```python
from build123d import *

# Parameters (mm, degrees)
SKETCH1_W                      = 5
SKETCH1_H                      = 25
BOSS_EXTRUDE1_DEPTH            = 10
BOSS_EXTRUDE2_DEPTH            = 2.5
BOSS_EXTRUDE3_START            = 2.5
BOSS_EXTRUDE3_DEPTH            = 2.5
BOSS_EXTRUDE4_DEPTH            = 5
DRAFT1_ANGLE                   = 60
DRAFT2_ANGLE                   = -10
SKETCH6_W                      = 5
SKETCH6_H                      = 15
SKETCH7_W                      = 5
SKETCH7_H                      = 15
SKETCH8_W                      = 5
SKETCH8_H                      = 25
F_10_0_10_DIAMETER_HOLE1_D     = 10
F_10_0_10_DIAMETER_HOLE1_DEPTH = 23.832037061
FILLET1_R                      = 5
FILLET2_R                      = 20


with BuildPart() as part:
    # Sketch1 → Revolve1 (revolve)
    with BuildSketch(Plane(origin=(0, -7.5, 0), x_dir=(1, 0, 0), z_dir=(0, 1, 0))):
        with Locations((-5.811233855, 90.876419512)):
            Rectangle(SKETCH1_W, SKETCH1_H)
    revolve(axis=Axis((-8.311233855, -7.5, -103.376419512), (0, 0, 1)))

    # Sketch2 → Boss-Extrude1 (add)
    with BuildSketch(Plane(origin=(0, -2.5, 0), x_dir=(1, 0, 0), z_dir=(0, 1, 0))):
        with BuildLine():
            Line((-20.904218066, -4.060593221), (-17.745761276, -10))
            ThreePointArc((-17.745761276, -10), (-16.42436709, -8.86625844), (-15.571850751, -7.348145002))
            Line((-15.571850751, -7.348145002), (-13.235172111, -0.671920317))
            ThreePointArc((-13.235172111, -0.671920317), (-13.124251068, -0.312083076), (-13.040724348, 0.055081199))
            ThreePointArc((-13.040724348, 0.055081199), (-9.034250588, -1.999882688), (-5, 0))
            ThreePointArc((-5, 0), (-1.464466094, 1.464466094), (0, 5))
            Line((0, 5), (0, 35))
            ThreePointArc((0, 35), (-10.533604853, 36.723434751), (-20.057952451, 41.541511272))
            Line((-20.057952451, 41.541511272), (5.197843412, 71.090018979))
            Line((5.197843412, 71.090018979), (8.982632418, 71.090018979))
            Line((8.982632418, 71.090018979), (8.982632418, 78.376419512))
            Line((8.982632418, 78.376419512), (-8.311233855, 78.376419512))
            Line((-8.311233855, 78.376419512), (-41.017367582, 78.376419512))
            Line((-41.017367582, 78.376419512), (-54.819345863, 40.83303933))
            Line((-54.819345863, 40.83303933), (-54.896976862, 16.766177236))
            ThreePointArc((-54.896976862, 16.766177236), (-54.712461515, 16.524099343), (-54.430876141, 16.639673113))
            Line((-54.430876141, 16.639673113), (-49.872077715, 24.477250263))
            Line((-49.872077715, 24.477250263), (-8.967847829, 0.684930874))
            Line((-8.967847829, 0.684930874), (-28.967743782, 0.74944331))
            Line((-28.967743782, 0.74944331), (-28.987601327, -5.406715976))
            ThreePointArc((-28.987601327, -5.406715976), (-28.311946244, -7.932877153), (-26.453503439, -9.772494077))
            Line((-26.453503439, -9.772494077), (-20.904218066, -4.060593221))
        make_face()
    extrude(amount=-BOSS_EXTRUDE1_DEPTH)

    # Sketch3 → Boss-Extrude2 (add)
    with BuildSketch(Plane.XZ.offset(12.5)):
        with BuildLine():
            Line((-20.904218066, 4.060593221), (-17.745761276, 10))
            ThreePointArc((-17.745761276, 10), (-16.42436709, 8.86625844), (-15.571850751, 7.348145002))
            Line((-15.571850751, 7.348145002), (-13.235172111, 0.671920317))
            ThreePointArc((-13.235172111, 0.671920317), (-13.124251068, 0.312083076), (-13.040724348, -0.055081199))
            ThreePointArc((-13.040724348, -0.055081199), (-9.034250588, 1.999882688), (-5, 0))
            ThreePointArc((-5, 0), (-1.464466094, -1.464466094), (0, -5))
            Line((0, -5), (0, -35))
            ThreePointArc((0, -35), (-10.533604853, -36.723434751), (-20.057952451, -41.541511272))
            Line((-20.057952451, -41.541511272), (5.197843412, -71.090018979))
            Line((5.197843412, -71.090018979), (8.982632418, -71.090018979))
            Line((8.982632418, -71.090018979), (8.982632418, -78.376419512))
            Line((8.982632418, -78.376419512), (-41.017367582, -78.376419512))
            Line((-41.017367582, -78.376419512), (-54.819345863, -40.83303933))
            Line((-54.819345863, -40.83303933), (-54.896976862, -16.766177236))
            ThreePointArc((-54.896976862, -16.766177236), (-54.712461515, -16.524099343), (-54.430876141, -16.639673113))
            Line((-54.430876141, -16.639673113), (-49.872077715, -24.477250263))
            Line((-49.872077715, -24.477250263), (-8.967847829, -0.684930874))
            Line((-8.967847829, -0.684930874), (-28.967743782, -0.74944331))
            Line((-28.967743782, -0.74944331), (-28.987601327, 5.406715976))
            ThreePointArc((-28.987601327, 5.406715976), (-28.311946244, 7.932877153), (-26.453503439, 9.772494077))
            Line((-26.453503439, 9.772494077), (-20.904218066, 4.060593221))
        make_face()
    extrude(amount=BOSS_EXTRUDE2_DEPTH)

    # Sketch4 → Boss-Extrude3 (add)
    with BuildSketch(Plane(origin=(0, -2.5, 0), x_dir=(-1, 0, 0), z_dir=(0, 1, 0)).offset(BOSS_EXTRUDE3_START)):
        with BuildLine():
            Line((20.904218066, 4.060593221), (26.453503439, 9.772494077))
            ThreePointArc((26.453503439, 9.772494077), (28.311946244, 7.932877153), (28.987601327, 5.406715976))
            Line((28.987601327, 5.406715976), (28.967743782, -0.74944331))
            Line((28.967743782, -0.74944331), (8.967847829, -0.684930874))
            Line((8.967847829, -0.684930874), (49.872077715, -24.477250263))
            Line((49.872077715, -24.477250263), (54.430876141, -16.639673113))
            ThreePointArc((54.430876141, -16.639673113), (54.712461515, -16.524099343), (54.896976862, -16.766177236))
            Line((54.896976862, -16.766177236), (54.819345863, -40.83303933))
            Line((54.819345863, -40.83303933), (41.017367582, -78.376419512))
            Line((41.017367582, -78.376419512), (-8.982632418, -78.376419512))
            Line((-8.982632418, -78.376419512), (-8.982632418, -71.090018979))
            Line((-8.982632418, -71.090018979), (-5.197843412, -71.090018979))
            Line((-5.197843412, -71.090018979), (20.057952451, -41.541511272))
            ThreePointArc((20.057952451, -41.541511272), (10.533604853, -36.723434751), (0, -35))
            Line((0, -35), (0, -5))
            ThreePointArc((0, -5), (1.464466094, -1.464466094), (5, 0))
            ThreePointArc((5, 0), (9.034250588, 1.999882688), (13.040724348, -0.055081199))
            ThreePointArc((13.040724348, -0.055081199), (13.124251068, 0.312083076), (13.235172111, 0.671920317))
            Line((13.235172111, 0.671920317), (15.571850751, 7.348145002))
            ThreePointArc((15.571850751, 7.348145002), (16.42436709, 8.86625844), (17.745761276, 10))
            Line((17.745761276, 10), (20.904218066, 4.060593221))
        make_face()
    extrude(amount=-BOSS_EXTRUDE3_DEPTH)

    # Sketch5 → Boss-Extrude4 (add)
    with BuildSketch(Plane.XY.offset(-103.376419512)):
        Polygon((-3.012739699, 4.048494156), (-14.561233855, 8.832037061), (-26.109728012, 4.048494156), (-30.893270916, -7.5), (-26.109728012, -19.048494156), (-14.561233855, -23.832037061), (-3.012739699, -19.048494156), (1.770803206, -7.5), align=None)
    extrude(amount=-BOSS_EXTRUDE4_DEPTH)

    # Draft1
    draft1_faces = [part.faces().sort_by_distance(p)[0] for p in [
        (-18.967795805, -7.5, -0.717187092),
    ]]
    draft(draft1_faces, Plane(origin=(-28.967743782, -12.5, -0.74944331), x_dir=(0.0032256218002524395, 0, -0.9999947976684688), z_dir=(-0.9999947976684688, 0, -0.0032256218002524395)), DRAFT1_ANGLE)

    # Draft2
    draft2_faces = [part.faces().sort_by_distance(p)[0] for p in [
        (8.982632418, -7.5, -74.733219246),
    ]]
    draft(draft2_faces, Plane(origin=(-8.311233855, -12.5, -78.376419512), x_dir=(-1, 0, 0), z_dir=(0, 0, -1)), DRAFT2_ANGLE)

    # Sketch6 → Cut-Revolve1 (revolve, cut)
    with BuildSketch(Plane.XY.offset(7)):
        with Locations((-19.5, -7.5)):
            Rectangle(SKETCH6_W, SKETCH6_H)
    revolve(axis=Axis((-22, 0, 7), (0, -1, 0)), mode=Mode.SUBTRACT)

    # Sketch7 → Cut-Revolve2 (revolve, cut)
    with BuildSketch(Plane(origin=(0, 0, -3), x_dir=(-1, 0, 0), z_dir=(0, 0, -1))):
        with Locations((6.5, -7.5)):
            Rectangle(SKETCH7_W, SKETCH7_H)
    revolve(axis=Axis((-9, -15, -3), (0, 1, 0)), mode=Mode.SUBTRACT)

    # Sketch8 → Revolve2 (revolve)
    with BuildSketch(Plane(origin=(0, -7.5, 0), x_dir=(1, 0, 0), z_dir=(0, 1, 0))):
        with Locations((-18.311233855, 90.876419512)):
            Rectangle(SKETCH8_W, SKETCH8_H)
    revolve(axis=Axis((-20.811233855, -7.5, -103.376419512), (0, 0, 1)))

    # Sketch9 → Revolve3 (revolve)
    with BuildSketch(Plane(origin=(0, -7.5, 0), x_dir=(1, 0, 0), z_dir=(0, 1, 0))):
        Polygon((-51.129054889, 22.316230044), (-52.386032062, 20.155209826), (-26.453789436, 5.071483748), (-25.196812263, 7.232503967), align=None)
    revolve(axis=Axis((-53.325247092, -7.5, -20.701512837), (0.8644080875330462, 0, 0.502790869256256)))

    # Ø10.0 (10) Diameter Hole1
    with Locations(Plane(origin=(0, -15, 0), x_dir=(-1, 0, 0), z_dir=(0, -1, 0))):
        with Locations((-0.318427602, 69.998551454)):
            Hole(F_10_0_10_DIAMETER_HOLE1_D / 2, depth=F_10_0_10_DIAMETER_HOLE1_DEPTH)

    # Chamfer1
    # the kernel refuses this chamfer: 0.262951912, 0.262770817 mm, written as the material it takes off along each edge
    with BuildSketch(Plane(origin=(-5, -15.679311202, 0), x_dir=(0.9996632496701223, 4.862291359988254e-15, -0.02594970633688609), z_dir=(0, 1, 0))) as chamfer1_piece_1:
        with BuildLine():
            Line((0.259497063, 0), (0.159812325, 0.213399124))
            ThreePointArc((0.159812325, 0.213399124), (0.082816569, 0.107621918), (0, 0))
            ThreePointArc((0, 0), (0.131972937, -0.001683257), (0.259497063, 0))
        make_face()
    extrude(amount=16.358622404, mode=Mode.SUBTRACT)

    # Fillet1
    fillet1_edges = [part.edges().sort_by_distance(p)[0] for p in [
        (-28.967743782, -7.5, -0.74944331),
        (8.982632418, -7.5, -78.376419512),
    ]]
    fillet(fillet1_edges, radius=FILLET1_R)

    # Fillet2
    fillet2_edges = [part.edges().sort_by_distance(p)[0] for p in [
        (-41.017367582, -7.5, -78.376419512),
        (-54.819345863, -7.5, -40.83303933),
    ]]
    fillet(fillet2_edges, radius=FILLET2_R)


solid = part.part
```
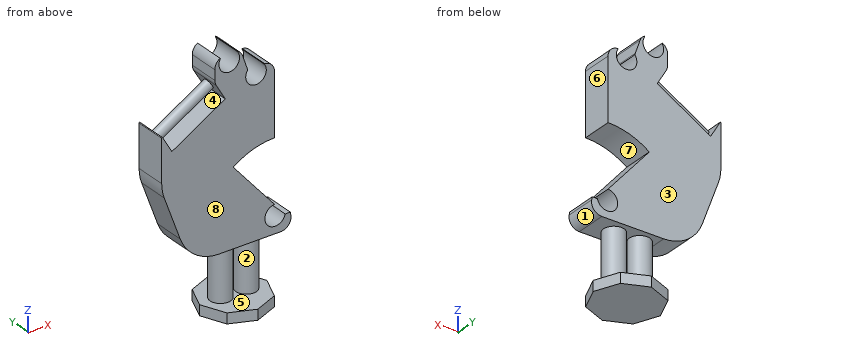
Input: part model. Units: mm. Frame: model coordinates. Face numbers are marked on the shaded views. A direction names the side the tool comes from. Coordinates: 2 decimals unless noted, no trailing zeros. Write each loop counter-clockwise with the first axis right and the second up, starting at its lowest first coordinate (ties: lowest second). Pieces come first, ordered by that corner, then holes.
1) Material intervals for line 1 along Y through (x, z) = (-44, -47); line 2 along X through (y, z) = (-12.5, -34.5); line 3 along Z through (x, y) = (-3, -11.5), sorted ascending.
2) Section D-D on y = -17.5. Output: boundary loops of the cut face in (x, z), and give its area (3 significant figures).
3) Section A-A on z = -93. Output: boundary loops of the cut face in (x, y).
4) Pin query (flat end, axial travel): pin 1 Ø5 at (y, z) = (-4.5, -31.5) entering from -X; pin 2 Ø8 at (y, z) = (-4, -14.5) entering from +X; pin 3 Ø19 at (x, z) = (-22.5, -21.5) entering from +Y; pin 4 Ø9 at (x, z) = (0.32, -70) entering from -Y. Return the tip coordinate at first contact, or that it passes through.
5) Mould query, pull axis X, two halves, no side actions, for the marked faces 1, 2, 3 and 4. Classes: pulls with the +X half, pulls with the -X half, needs draft (parallel to the pull), parting line crosses it, or undercut.
6) Section B-B on x = -9. Output: boundary loops of the cut face in (y, z), and give its area (3 significant figures).
7) Set-up query: the marked faces 5, 6, 7 and 8. Return all of +Z, -Z, +X, -X, +Y, -Y with unobstructed straight access to the full face (end or side cutting, diameter ignored); none if empty.
8) Section C-C on x = -22. Output: boundary loops of the cut face in (y, z).
Check result:
1. line 1: y = -15 to 0
1. line 2: x = -54.84 to 0
1. line 3: z = -108.38 to -103.38, -78.38 to -73.74, -66.26 to -61.5, -35.16 to -0.42
2. outline: (-26.75, -108.38) - (-2.37, -108.38) - (-2.37, -103.38) - (-26.75, -103.38) - close
2. area: 122 mm2
3. outline: circle Ø10 at (-20.81, -7.5); circle Ø10 at (-8.31, -7.5)
4. pin 1: stops at x = -54.86
4. pin 2: stops at x = 0
4. pin 3: stops at y = 0
4. pin 4: passes through
5. face 1: pulls with the +X half
5. face 2: undercut
5. face 3: needs draft
5. face 4: undercut
6. outline: (-21.53, -108.38) - (6.53, -108.38) - (6.53, -103.38) - (-2.55, -103.38) - (-2.55, -78.38) - (0, -78.38) - (0, -54.48) - (-15, -54.48) - (-15, -78.38) - (-12.45, -78.38) - (-12.45, -103.38) - (-21.53, -103.38) - close; (-15, -36.26) - (0, -36.26) - (0, -8) - (-15, -8) - close
6. area: 1,170 mm2
7. face 5: none
7. face 6: +Z, +X, +Y, -Y
7. face 7: +X, +Y, -Y
7. face 8: +Z, +X, -X, -Y
8. outline: (-20.75, -108.38) - (5.75, -108.38) - (5.75, -103.38) - (-2.64, -103.38) - (-2.64, -78.38) - (0, -78.38) - (0, 2) - (-15, 2) - (-15, -78.38) - (-12.36, -78.38) - (-12.36, -103.38) - (-20.75, -103.38) - close
